Build history of the part. All positions in model axes, mm. Face numbers are marked on the shaded views. A direction names the side the tool comes from. Give positions to 0.01 mm unless a question says otherwise; leave off trailing zeros. Loops run counter-clockwise (first coordinate to the right, second up) from the corner with the lowest first, then second, coordinate; pieces in that order, holes last. Notation, with made-up numbers: (-3.75, -38) -> (31.25, -38) arc R28 ccw to (31.25, -12) -> close; hole circle Ø6 at (42.5, -28). An arc over 180 degrees is marked (long way). Answer as a JSON object with one key per item and string values. Group by question number.
Q1. Band-saw the part on D-D, the plane x = -41.5. Write the cut outline in (y, z).
Q2. Band-saw the part on B-B, the plane y = -45. Write the cut outline in (x, z).
Q3. Tool access for the marked faces 3, 4, 5, 6 and 7: list every direction of +Z, -Z, +X, -X, +Y, -Y with a clear straight run to the whole face (end or side of a thin tool).
Q4. Band-saw the part on C-C, the plane x = -65. Write the cut outline in (y, z).
Q5. Band-saw the part on A-A, the plane z = -18.5. Write the cut outline in (x, y), plus the area to 3 significant figures.
Q6. Two-plate mould, pull along X, no slides. Class the marked faces 1 and 2: pulls with the +X half, pulls with the -X half, needs draft (parallel to the pull), parting line crosses it, or undercut.
Q7. Drop flat-ended pins along their axis: pin 1 (11 mm diameter, centred on x = -8.5, y = -43.5, fed in from +Z); pin 2 (0.9 mm diameter, centred on x = -26.5, y = -32.5, fed in from +Z); pin 3 (6.5 mm diameter, centred on x = 27, y = -27.5, fed in from +Z); pin 4 (6.5 mm diameter, centred on x = -65, y = -45, fed in from +Z). Give the stop position or say it passes through.
Q8. Wall check: probe 1 along Y at (x, z) = (-65, -42.5); probe 2 along Z at (x, y) = (-4, -5.5); probe 3 along X at (y, z) = (29, -30). Give the ranges that are in metal, low to high. Write a range as from..to.
from build123d import *

# Parameters (mm, degrees)
F0_W      = 10
F0_H      = 10
F1_DEPTH  = 65
F4_DEPTH  = 8
F5_W      = 140
F5_H      = 83
F6_DEPTH  = 4
F7_R      = 3
F7_R_2    = 1.5
F8_DEPTH  = 10.5
F9_R      = 3.5
F10_DEPTH = 70


with BuildPart() as f1:
    # F0 (on Top) → F1 (new body)
    with BuildSketch(Plane.XY):
        with Locations((-65, 28)):
            Rectangle(F0_W, F0_H)
        with Locations((65, 28)):
            Rectangle(F0_W, F0_H)
        with Locations((-65, -45)):
            Rectangle(F0_W, F0_H)
        with Locations((65, -45)):
            Rectangle(F0_W, F0_H)
    extrude(amount=-F1_DEPTH)

    # F3 (on offset) → F4 (join)
    with BuildSketch(Plane.XY.offset(-65)):
        Polygon((-70, -40), (-70, -50), (-60, -50), (60, -50), (70, -50), (70, -40), (70, 23), (60, 23), (60, -40), (-60, -40), (-60, 23), (-70, 23), align=None)
        Polygon((-70, 33), (-70, 23), (-60, 23), (60, 23), (70, 23), (70, 33), align=None)
    extrude(amount=F4_DEPTH)

    # F5 (on offset) → F6 (join)
    with BuildSketch(Plane.XY.offset(-65)):
        with Locations((0, -8.5)):
            Rectangle(F5_W, F5_H)
    extrude(amount=F6_DEPTH)

    # F7 (on offset) → F8 (join)
    with BuildSketch(Plane.XY.offset(-65)):
        with Locations((-24.34509, 15.832442)):
            Circle(F7_R)
        with Locations((-24.34509, 15.832442)):
            Circle(F7_R_2, mode=Mode.SUBTRACT)
        with Locations((26.337272, 0.330886)):
            Circle(F7_R)
        with Locations((26.337272, 0.330886)):
            Circle(F7_R_2, mode=Mode.SUBTRACT)
        with Locations((26.613058, -27.667755)):
            Circle(F7_R)
        with Locations((26.613058, -27.667755)):
            Circle(F7_R_2, mode=Mode.SUBTRACT)
        with Locations((-25.65, -32.65)):
            Circle(F7_R)
        with Locations((-25.65, -32.65)):
            Circle(F7_R_2, mode=Mode.SUBTRACT)
    extrude(amount=F8_DEPTH)

    # F9 (on Top) → F10 (cut)
    with BuildSketch(Plane.XY):
        with Locations((-65, 28)):
            Circle(F9_R)
        with Locations((-65, -45)):
            Circle(F9_R)
        with Locations((65, -45)):
            Circle(F9_R)
        with Locations((65, 28)):
            Circle(F9_R)
    extrude(amount=-F10_DEPTH, mode=Mode.SUBTRACT)


solid = f1.part
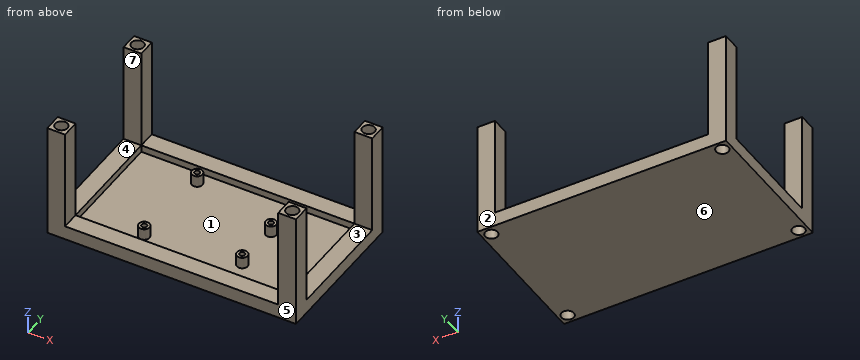
Worked answers:
{
 "1": {"outline": "(-50, -65) -> (33, -65) -> (33, -57) -> (23, -57) -> (23, -61) -> (-40, -61) -> (-40, -57) -> (-50, -57) -> close"},
 "2": {"outline": "(-70, -65) -> (-68.5, -65) -> (-68.5, 0) -> (-70, 0) -> close; (-61.5, -65) -> (61.5, -65) -> (61.5, 0) -> (60, 0) -> (60, -57) -> (-60, -57) -> (-60, 0) -> (-61.5, 0) -> close; (68.5, -65) -> (70, -65) -> (70, 0) -> (68.5, 0) -> close"},
 "3": {"face 3": "+Z, +X", "face 4": "+Z, -X", "face 5": "+Z, -Z, +X, -X, -Y", "face 6": "-Z, +X, -X, +Y, -Y", "face 7": "+Z, +X, -X"},
 "4": {"outline": "(-50, -65) -> (-48.5, -65) -> (-48.5, 0) -> (-50, 0) -> close; (-41.5, -65) -> (24.5, -65) -> (24.5, 0) -> (23, 0) -> (23, -57) -> (-40, -57) -> (-40, 0) -> (-41.5, 0) -> close; (31.5, -65) -> (33, -65) -> (33, 0) -> (31.5, 0) -> close"},
 "5": {"outline": "(-70, -50) -> (-60, -50) -> (-60, -40) -> (-70, -40) -> close; (-70, 23) -> (-60, 23) -> (-60, 33) -> (-70, 33) -> close; (60, -50) -> (70, -50) -> (70, -40) -> (60, -40) -> close; (60, 23) -> (70, 23) -> (70, 33) -> (60, 33) -> close; hole circle Ø7 at (-65, -45); hole circle Ø7 at (-65, 28); hole circle Ø7 at (65, -45); hole circle Ø7 at (65, 28)", "area": "246 mm2"},
 "6": {"face 1": "undercut", "face 2": "needs draft"},
 "7": {"pin 1": "z = -57", "pin 2": "z = -61", "pin 3": "z = -54.5", "pin 4": "through"},
 "8": {"probe 1": "-50..-48.5, -41.5..-40, 23..24.5, 31.5..33", "probe 2": "-65..-61", "probe 3": "-70..-68.35, -61.65..-60, 60..61.65, 68.35..70"}
}
